from build123d import *

# Parameters (mm, degrees)
F0_W      = 50.8
F0_H      = 50.8
F1_DEPTH  = 50.8
F2_R      = 3.81
F3_DEPTH  = 2.54
F4_R      = 3.81
F5_DEPTH  = 2.54
F6_R      = 3.81
F7_DEPTH  = 2.54
F8_R      = 3.81
F9_DEPTH  = 2.54
F10_R     = 3.81
F11_DEPTH = 2.54
F12_R     = 3.81
F13_DEPTH = 2.54


with BuildPart() as f1:
    # F0 (on Front) → F1 (new body)
    with BuildSketch(Plane.XZ):
        with Locations((-50.8, -50.8)):
            Rectangle(F0_W, F0_H)
    extrude(amount=F1_DEPTH)

    # F2 (on face) → F3 (cut)
    with BuildSketch(Plane(origin=(-76.2, 0, 0), x_dir=(0, -1, 0), z_dir=(-1, 0, 0))):
        with Locations((25.4, -50.8)):
            Circle(F2_R)
    extrude(amount=-F3_DEPTH, mode=Mode.SUBTRACT)

    # F4 (on face) → F5 (cut)
    with BuildSketch(Plane.YZ.offset(-25.4)):
        with Locations((-12.7, -63.5)):
            Circle(F4_R)
        with Locations((-38.1, -38.1)):
            Circle(F4_R)
    extrude(amount=-F5_DEPTH, mode=Mode.SUBTRACT)

    # F6 (on face) → F7 (cut)
    with BuildSketch(Plane.XZ.offset(50.8)):
        with Locations((-50.8, -50.8)):
            Circle(F6_R)
        with Locations((-64.847043, -36.752957)):
            Circle(F6_R)
        with Locations((-36.675387, -64.77)):
            Circle(F6_R)
    extrude(amount=-F7_DEPTH, mode=Mode.SUBTRACT)

    # F8 (on face) → F9 (cut)
    with BuildSketch(Plane(origin=(0, 0, 0), x_dir=(-1, 0, 0), z_dir=(0, 1, 0))):
        with Locations((38.1, -38.1)):
            Circle(F8_R)
        with Locations((63.5, -38.1)):
            Circle(F8_R)
        with Locations((38.1, -63.5)):
            Circle(F8_R)
        with Locations((63.5, -63.5)):
            Circle(F8_R)
    extrude(amount=-F9_DEPTH, mode=Mode.SUBTRACT)

    # F10 (on face) → F11 (cut)
    with BuildSketch(Plane.XY.offset(-25.4)):
        with Locations((-63.5, -12.7)):
            Circle(F10_R)
        with Locations((-38.1, -12.7)):
            Circle(F10_R)
        with Locations((-63.5, -38.1)):
            Circle(F10_R)
        with Locations((-38.1, -38.1)):
            Circle(F10_R)
        with Locations((-50.8, -25.4)):
            Circle(F10_R)
    extrude(amount=-F11_DEPTH, mode=Mode.SUBTRACT)

    # F12 (on face) → F13 (cut)
    with BuildSketch(Plane(origin=(0, 0, -76.2), x_dir=(1, 0, 0), z_dir=(0, 0, -1))):
        with Locations((-60.96, 25.4)):
            Circle(F12_R)
        with Locations((-60.96, 38.1)):
            Circle(F12_R)
        with Locations((-60.96, 12.7)):
            Circle(F12_R)
        with Locations((-40.64, 12.7)):
            Circle(F12_R)
        with Locations((-40.64, 25.4)):
            Circle(F12_R)
        with Locations((-40.64, 38.1)):
            Circle(F12_R)
    extrude(amount=-F13_DEPTH, mode=Mode.SUBTRACT)


solid = f1.part
The listing builds one solid part. Answer for the finished solid, in the listing's coordinates (mm). A direction names the side the tool comes from. Coordinates: 2 decimals unless noted, no trailing zeros. Write each loop counter-clockwise with the first axis right and the second up, starting at its lowest first coordinate (ties: lowest second). Pieces come first, ordered by that corner, then holes. Notation, with made-up numbers: (-9.75, 31) -> (45.25, 31) arc R12 ccw to (45.25, 47) -> close; hole circle Ø10 at (7, 8). An arc over 180 degrees is marked (long way). One line per question, with ' | ' between items.
1. Which of the six approach directions +Z, -Z, +X, -X, +Y, -Y give full straight-line access (tool end or side, diameter ignored) to faces 4 (the cylindrical face through (-39.7, -49.55, -67.09)), 5 (the cylindrical face through (-59.2, -34.72, -74.95)), 6 (the flat face through (-38, -13, -27.94)), 7 (the flat face through (-27.94, -38, -38))?
Verdict:
face 4: -Y | face 5: -Z | face 6: +Z | face 7: +X
2. Section D-D (z = -38.1) is taken. Determine the outline of the cut face in (x, y), and give its area (3 significant figures).
Verdict:
outline: (-76.2, -50.8) -> (-68.41, -50.8) -> (-68.41, -48.26) -> (-61.28, -48.26) -> (-61.28, -50.8) -> (-25.4, -50.8) -> (-25.4, -41.91) -> (-27.94, -41.91) -> (-27.94, -34.29) -> (-25.4, -34.29) -> (-25.4, 0) -> (-34.29, 0) -> (-34.29, -2.54) -> (-41.91, -2.54) -> (-41.91, 0) -> (-59.69, 0) -> (-59.69, -2.54) -> (-67.31, -2.54) -> (-67.31, 0) -> (-76.2, 0) -> close | area: 2,500 mm^2
3. For a pull along Y with two mould halves and no side action, classify faces 1 (the cylindrical face through (-43.66, -35.78, -74.95)), 2 (the flat face through (-65, -48.26, -37)), 3 (the cylindrical face through (-62.67, -1.25, -67.22)) as released by +Y, released by -Y, zero draft, split by the parting line, or undercut.
Verdict:
face 1: undercut | face 2: released by -Y | face 3: zero draft
4. Section C-C (x = -50.8) is taken. Determine the outline of the cut face in (y, z), and give its area (3 significant figures).
Verdict:
outline: (-50.8, -76.2) -> (0, -76.2) -> (0, -25.4) -> (-21.59, -25.4) -> (-21.59, -27.94) -> (-29.21, -27.94) -> (-29.21, -25.4) -> (-50.8, -25.4) -> (-50.8, -46.99) -> (-48.26, -46.99) -> (-48.26, -54.61) -> (-50.8, -54.61) -> close | area: 2,540 mm^2
5. Section B-B (z = -50.8) is taken. Determine the outline of the cut face in (x, y).
Verdict:
outline: (-76.2, -50.8) -> (-54.61, -50.8) -> (-54.61, -48.26) -> (-46.99, -48.26) -> (-46.99, -50.8) -> (-25.4, -50.8) -> (-25.4, 0) -> (-76.2, 0) -> (-76.2, -21.59) -> (-73.66, -21.59) -> (-73.66, -29.21) -> (-76.2, -29.21) -> close
6. Given pin 1 Ø4.5 at (x, y) = (-60.96, -12.7) entering from -Z; pin 2 Ø6 at (x, z) = (-38.5, -38) entering from +Y; pin 3 Ø9 at (x, z) = (-64.85, -36.75) entering from +Y; pin 4 Ø6 at (x, z) = (-51, -50.5) entering from -Y, each flat-ended and moving along its own axis, determine where each tip first touches the part or whether it passes through.
Verdict:
pin 1: stops at z = -73.66 | pin 2: stops at y = -2.54 | pin 3: stops at y = 0 | pin 4: stops at y = -48.26
7. Straight lines are drawn through the part: line 1 (X direction, y = -38.1, z = -75.1); line 2 (Y direction, x = -60.96, z = -74.35); line 3 (Y direction, x = -38.1, z = -27.4). For each, find the intervals that lie inside material, in ascending order.
Verdict:
line 1: x = -76.2 to -64.77, -57.15 to -44.45, -36.83 to -25.4 | line 2: y = -50.8 to -41.91, -34.29 to -29.21, -21.59 to -16.51, -8.89 to 0 | line 3: y = -50.8 to -41.91, -34.29 to -16.51, -8.89 to 0
8. Section A-A (y = -25.4) is taken. Determine the outline of the cut face in (x, z).
Verdict:
outline: (-76.2, -76.2) -> (-64.77, -76.2) -> (-64.77, -73.66) -> (-57.15, -73.66) -> (-57.15, -76.2) -> (-44.45, -76.2) -> (-44.45, -73.66) -> (-36.83, -73.66) -> (-36.83, -76.2) -> (-25.4, -76.2) -> (-25.4, -25.4) -> (-46.99, -25.4) -> (-46.99, -27.94) -> (-54.61, -27.94) -> (-54.61, -25.4) -> (-76.2, -25.4) -> (-76.2, -46.99) -> (-73.66, -46.99) -> (-73.66, -54.61) -> (-76.2, -54.61) -> close
